Autodesk Inventor part; units mm, degrees
ref_plane "YZ Plane" through (0, 0, 0) normal (1, 0, 0) x (0, 1, 0)
ref_plane "XZ Plane" through (0, 0, 0) normal (0, 1, 0) x (-1, 0, 0)
ref_plane "XY Plane" through (0, 0, 0) normal (0, 0, 1) x (1, 0, 0)
sketch "Sketch2" plane through (0, 0, 0) normal (0, 1, 0) x (-1, 0, 0)
  line L0 (-16, 16) -> (16, 16)
  line L1 (16, 16) -> (16, -16)
  line L2 (16, -16) -> (-16, -16)
  line L3 (-16, -16) -> (-16, 16)
  point P0 (0, 0)
  point P1 (0, 16)
  point P2 (-16, 0)
  dimension "d0" = 32
  dimension "d1" = 32
extrude "Extrusion1" add sketch "Sketch2" along normal blind 3.2
sketch "Sketch3" plane through (0, 0, 0) normal (0, -1, 0) x (1, 0, 0)
  line L0 (-16, 16) -> (-16, -16)
  line L1 (-14.4, 14.4) -> (14.4, 14.4)
  line L2 (14.4, 14.4) -> (14.4, -14.4)
  line L3 (14.4, -14.4) -> (-14.4, -14.4)
  line L4 (-14.4, -14.4) -> (-14.4, 14.4)
  circle A0 centre (-8, 0) radius 3.2569
  circle A1 centre (-8, 0) radius 2.4
  line L5 (-16, -16) -> (16, -16)
  circle A2 centre (0, 0) radius 1.6
  line L6 (16, -16) -> (16, 16)
  line L7 (-12, 0) -> (-4, 0) construction
  line L8 (-4, 0) -> (4, 0) construction
  line L9 (4, 0) -> (12, 0) construction
  circle A3 centre (-12, 12) radius 2.4 construction
  circle A4 centre (-12, -12) radius 2.4 construction
  circle A5 centre (12, -12) radius 2.4 construction
  circle A6 centre (12, 12) radius 2.4 construction
  line L10 (16, 16) -> (-16, 16)
  line L11 (-15.6, 15.6) -> (15.6, 15.6)
  line L12 (15.6, 15.6) -> (15.6, -15.6)
  line L13 (15.6, -15.6) -> (-15.6, -15.6)
  line L14 (-15.6, -15.6) -> (-15.6, 15.6)
  circle A7 centre (-12, 4) radius 2.4 construction
  point P0 (-14.4, 0)
  point P1 (0, 14.4)
  point P2 (0, 0)
  point P3 (0, 15.6)
  point P4 (-15.6, 0)
  dimension "d61" = 4.8
  dimension "d75" = 8
  dimension "d76" = 16
  dimension "d86" = 3.2
  dimension "d92" = 8
  dimension "d98" = 24
  dimension "d99" = 24
  dimension "d102" = 0.4
  dimension "d103" = 0.4
  dimension "d106" = 8
extrude "Extrusion2" cut sketch "Sketch3" against normal blind 1.6 contours L1 L2 L3 L4 | A0 | A1 | A2
extrude "Extrusion7" cut sketch "Sketch3" against normal blind 0.4 contours L10 L6 L5 L0
extrude "Extrusion6" add sketch "Sketch3" against normal up to next contours A0
pattern_linear "Rectangular Pattern3" count 3 spacing 8 along (1, 0, 0) count 3 spacing 8 along (0, 0, -1) of "Extrusion6" second direction both ways yes
fillet "Fillet1" radius 0.1 8 edges at (-16, 1.8, 16) (0, 3.2, 16) (-16, 3.2, 0) (16, 1.8, 16) (16, 3.2, 0) (0, 3.2, -16) (16, 1.8, -16) (-16, 1.8, -16)
sketch "Skizze10" plane through (0, 3.2, 0) normal (0, 1, 0) x (1, 0, 0)
  line L0 (-15.9, 15.9) -> (15.9, 15.9)
  line L1 (-16.3705, 16.4) -> (16.3705, 16.4) construction
  line L2 (16.3705, 16.4) -> (16.3705, -16.4) construction
  line L3 (16.3705, -16.4) -> (-16.3705, -16.4) construction
  line L4 (-16.3705, -16.4) -> (-16.3705, 16.4) construction
  point P0 (0, 0)
  point P1 (0, 16.4)
  point P2 (-16.3705, 0)
  dimension "d123" = 0.5
decal "Aufkleber1"
equation "\"d4\" = 0.333333 * lh"
equation "\"d61\" = kd"
equation "\"d75\" = lu"
equation "\"d76\" = 2 * d75"
equation "\"d86\" = pd"
equation "\"d92\" = lu"
equation "\"d98\" = d99"
equation "\"d99\" = 3 * d75"
equation "\"d102\" = gw"
equation "\"d103\" = gw"
equation "\"d106\" = lu"
equation "\"d11\" = 0.333333 * lh - topthk"
equation "\"d104\" = gh"
equation "\"d91\" = lu"
equation "\"d109\" = lu"
equation "\"d22\" = lf"
properties part number "42146_1751_1" material "ABS Plastic"
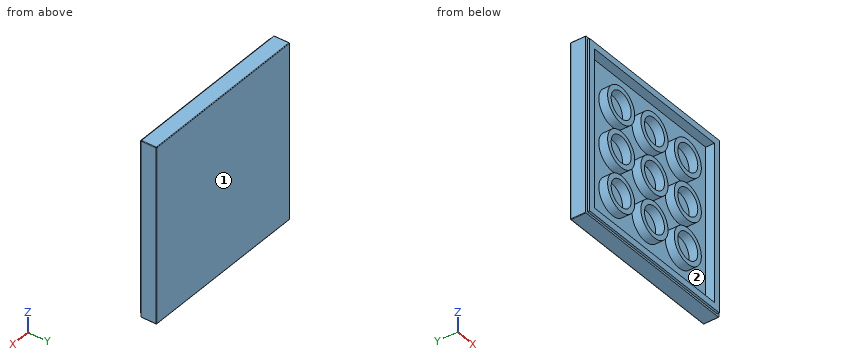
Verification items for the finished model (mm, model axes). Face numbers are marked on the shaded views. Coordinates: 2 decimals unless noted, no trailing zeros. Loops run counter-clockwise (first coordinate to the right, second up) from the corner with the lowest first, then second, coordinate; pieces in that order, holes last. Notation, with made-up numbers: (85, 67.25) -> (102, 67.25) arc R14 cw to (102, 86.25) -> close; hole circle Ø9 at (83, -15). An arc over 180 degrees is marked (long way). Answer as a JSON object with one key per item and string values. Group by question number.
Item 1: Sectioned sample at A-A on z = 12. Record the boundary of the cut face in (x, y).
Item 2: Mould release check, pull along Z, two halves, no side actions. Record for the marked faces 1 and 2: +Z half, -Z half, draft (parallel to the pull), parting line (faces both ways), or undercut.
Item 3: Depth check by flat-ended pin: pin 1 (4 mm diameter, centred on x = -8.5, z = 7.5, fed in from -Y); pin 2 (4.5 mm diameter, centred on x = 8, z = 8, fed in from -Y). Enter the tip coordinate at first touch or a pass-through.
Item 4: Scan lines: probe 1 along X at (y, z) = (0.3, -13.5); probe 2 along Y at (x, z) = (-8, -6.5); probe 3 along X at (y, z) = (1.1, 5.5). Record each from-to range of solid material in increasing order.
Item 5: Sectioned sample at B-B on x = 4. Record the boundary of the cut face in (y, z).
Evaluation:
{
 "1": {"outline": "(-16, 0.4) -> (-15.6, 0.4) -> (-15.6, 0) -> (-14.4, 0) -> (-14.4, 1.6) -> (14.4, 1.6) -> (14.4, 0) -> (15.6, 0) -> (15.6, 0.4) -> (16, 0.4) -> (16, 3.1) arc R0.1 ccw to (15.9, 3.2) -> (-15.9, 3.2) arc R0.1 ccw to (-16, 3.1) -> close"},
 "2": {"face 1": "draft", "face 2": "undercut"},
 "3": {"pin 1": "stops at y = 0", "pin 2": "stops at y = 1.6"},
 "4": {"probe 1": "x = -15.6 to -14.4, 14.4 to 15.6", "probe 2": "y = 1.6 to 3.2", "probe 3": "x = -16 to -14.4, -10.09 to -5.91, -2.09 to 2.09, 5.91 to 10.09, 14.4 to 16"},
 "5": {"outline": "(0, -15.6) -> (0.4, -15.6) -> (0.4, -16) -> (3.1, -16) arc R0.1 ccw to (3.2, -15.9) -> (3.2, 15.9) arc R0.1 ccw to (3.1, 16) -> (0.4, 16) -> (0.4, 15.6) -> (0, 15.6) -> (0, 14.4) -> (1.6, 14.4) -> (1.6, -14.4) -> (0, -14.4) -> close"}
}
